Could you check a few things on this model? Use its own coordinates, in mm. A direction names the side the tool comes from. Round coordinates to 2 decimals unless told otherwise and drop trailing zeros. Loops run counter-clockwise (first coordinate to the right, second up) from the corner with the lowest first, then second, coordinate; pieces in that order, holes last. Notation, with made-up numbers: (-6.5, 46) -> (28.5, 46) arc R20 ccw to (28.5, 57) -> close; hole circle Ø9 at (21.25, 19). An arc over 180 degrees is marked (long way). One line per item, written item: value.
```python
from build123d import *

# Parameters (mm, degrees)
SALIENTE_EXTRUIR1_DEPTH = 10
CORTAR_EXTRUIR1_DEPTH   = 113.828716794
CROQUIS5_R              = 3
CORTAR_EXTRUIR2_DEPTH   = 113.828716928


with BuildPart() as part:
    # Croquis1 → Revolución1 (revolve)
    with BuildSketch(Plane.XY):
        Polygon((0, 0), (-31.448700737, 77.838265751), (-24.977492281, 77.838265751), (0, 16.016802975), align=None)
    revolve(axis=Axis((0, 0, 0), (0, 1, 0)))

    # Croquis2 → Saliente-Extruir1 (add)
    with BuildSketch(Plane(origin=(0, 77.838265751, 0), x_dir=(1, 0, 0), z_dir=(0, 1, 0))):
        with BuildLine():
            Line((10, -22.888318432), (10, -29.816451466))
            ThreePointArc((10, -29.816451466), (0, -31.448700737), (-10, -29.816451466))
            Line((-10, -29.816451466), (-10, -22.888318432))
            ThreePointArc((-10, -22.888318432), (0, -24.977492281), (10, -22.888318432))
        make_face()
        with BuildLine():
            Line((10, 22.888318432), (10, 29.816451466))
            ThreePointArc((10, 29.816451466), (0, 31.448700737), (-10, 29.816451466))
            Line((-10, 29.816451466), (-10, 22.888318432))
            ThreePointArc((-10, 22.888318432), (0, 24.977492281), (10, 22.888318432))
        make_face()
    extrude(amount=SALIENTE_EXTRUIR1_DEPTH)

    # Croquis3 → Cortar-Extruir1 (cut, through all)
    with BuildSketch(Plane.XY.offset(32)):
        with BuildLine():
            Line((10, 87.838265751), (10, 77.838265751))
            ThreePointArc((10, 77.838265751), (7.071067812, 84.909333563), (0, 87.838265751))
            Line((0, 87.838265751), (10, 87.838265751))
        make_face()
    extrude(amount=-CORTAR_EXTRUIR1_DEPTH, mode=Mode.SUBTRACT)

    # Croquis5 → Cortar-Extruir2 (cut, through all)
    with BuildSketch(Plane.XY.offset(32)):
        with Locations((0, 82.338265751)):
            Circle(CROQUIS5_R)
        with BuildLine():
            Line((-10, 77.838265751), (-10, 87.838265751))
            Line((-10, 87.838265751), (0, 87.838265751))
            ThreePointArc((0, 87.838265751), (-7.071067812, 84.909333563), (-10, 77.838265751))
        make_face()
    extrude(amount=-CORTAR_EXTRUIR2_DEPTH, mode=Mode.SUBTRACT)


solid = part.part
```
Item 1: Will these pins go through, and if not, where does the flat tip stop? pin 1 Ø4 at (x, z) = (19.5, 7) entering from -Y; pin 2 Ø2 at (x, z) = (-7, 8.5) entering from -Y; pin 3 Ø17 at (x, z) = (20, 11.5) entering from +Y; pin 4 Ø9.5 at (x, y) = (0, 82.34) entering from +Z.
Output:
pin 1: stops at y = 46.33
pin 2: stops at y = 24.78
pin 3: stops at y = 77.84
pin 4: stops at z = 31.45
Item 2: If we mould it in two halves opening along X, with no side actions, what happens to faces 1 (the face through (-9.1, 39.63, 2.87)), 2 (the face through (-2.117, 79.435, -31.377)), 3 (the face through (-25.4, 77.838, 2.3))? For each: released by +X, released by -X, zero draft, split by the parting line, or undercut.
Output:
face 1: undercut
face 2: split by the parting line
face 3: zero draft
Item 3: If we section it at A-A on y = 51: List the corners of the cut face in (x, z) for me.
Output:
outline: circle Ø41.21 at (0, 0); hole circle Ø28.27 at (0, 0)
Item 4: If we section it at B-B on y = 12: List the corners of the cut face in (x, z) for me, plus the area to 3 significant figures.
Output:
outline: circle Ø9.7 at (0, 0)
area: 73.8 mm²
Item 5: For faces 4 (the face through (-2.43, 79.43, -24.86)), 5 (the face through (26, 77.838, 0)), 6 (the face through (-0.65, 79.41, -28.08)), which set-ups out of +Z, -Z, +X, -X, +Y, -Y let a thin tool reach every point of the face, with its end or its side?
Output:
face 4: +Y
face 5: +Z, -Z, +X, +Y
face 6: +Z, -Z
Item 6: I need wall thicknesses on line 1 (X direction, y = 77.5, z = 2.5); line 2 (X direction, y = 21.5, z = -0.5); line 3 (Y direction, x = 0, z = -27.25). Which ranges of each line are inside material? Lowest first, please. Write a range as from..to.
Output:
line 1: x = -31.21..-24.71, 24.71..31.21
line 2: x = -8.67..-2.16, 2.16..8.67
line 3: y = 67.45..79.34, 85.34..87.84
